```python
from build123d import *

# Parameters (mm, degrees)
F3_DEPTH  = 14
F5_DEPTH  = 5
F6_SIZE   = 2
F7_DEPTH  = 25
F9_DEPTH  = 51.6
F10_DEPTH = 1.1


# Not quite as in the source:
# - a feature names something its author has since deleted; it is built from what else it names


with BuildPart() as f3:
    # F2 (on line) → F3 (new body)
    with BuildSketch(Plane(origin=(0, 0, 0), x_dir=(0, 1, 0), z_dir=(0.984807753, 0, -0.1736481777))):
        with BuildLine():
            ThreePointArc((4.3133513652, 4.3133513652), (5.6356651483, 2.3343689374), (6.1, 0))
            ThreePointArc((6.1, 0), (-2.3343689374, -5.6356651483), (-4.3133513652, 4.3133513652))
            Line((-4.3133513652, 4.3133513652), (-6.4346717088, 6.4346717088))
            ThreePointArc((-6.4346717088, 6.4346717088), (-3.4824192345, -8.4073037459), (9.1, 0))
            ThreePointArc((9.1, 0), (8.4073037459, 3.4824192345), (6.4346717088, 6.4346717088))
            Line((6.4346717088, 6.4346717088), (4.3133513652, 4.3133513652))
        make_face()
    extrude(amount=F3_DEPTH)

    # F4 (on Front) → F5 (join, symmetric)
    with BuildSketch(Plane.XZ):
        Polygon((-0.9719453416, -8.4384017807), (-0.9719453416, -21.6384017807), (7.9780546584, -21.6384017807), (7.9780546584, -18.6384017807), (2.0280546584, -18.6384017807), (2.0280546584, -11.4384017807), (9.7280546584, -11.4384017807), (9.7280546584, -15.6384017807), (12.7280546584, -15.6384017807), (12.7280546584, -11.4438512443), (12.7280546584, -8.4384017807), align=None)
    extrude(amount=F5_DEPTH, both=True)

    # F6
    f6_edges = [f3.edges().sort_by_distance(p)[0] for p in [
        (9.728055, 0, -15.638402),
        (7.978055, 0, -18.638402),
    ]]
    chamfer(f6_edges, length=F6_SIZE)

    # F7 (add): a face of the model
    f7_faces = [f3.faces().sort_by_distance(p)[0] for p in [
        (-1.1008050308, 0, -6.2429755581),
    ]]
    extrude(f7_faces, amount=F7_DEPTH)

    # F8 (on face) → F9 (cut)
    with BuildSketch(Plane(origin=(-0.9719453416, 0, 0), x_dir=(0, -1, 0), z_dir=(-1, 0, 0))):
        with BuildLine():
            Line((22.6868242025, -11.5467039868), (22.6868242025, 11.5467039868))
            Line((22.6868242025, 11.5467039868), (-22.6868242025, 11.5467039868))
            Line((-22.6868242025, 11.5467039868), (-22.6868242025, -11.5467039868))
            Line((-22.6868242025, -11.5467039868), (-5, -11.5467039868))
            Line((-5, -11.5467039868), (-5, -8.4384017807))
            Line((-5, -8.4384017807), (-3.3040728779, -8.4384017807))
            add(Edge.make_bspline(
                [(-3.3040728779, -8.4384017807), (0, -9.7457887872), (3.3040728779, -8.4384017807)],
                knots=[2.7700160081, 2.7700160081, 2.7700160081, 3.5131692991, 3.5131692991, 3.5131692991], degree=2, weights=[1, 0.9317560477, 1]))
            Line((3.3040728779, -8.4384017807), (5, -8.4384017807))
            Line((5, -8.4384017807), (5, -11.5467039868))
            Line((5, -11.5467039868), (22.6868242025, -11.5467039868))
        make_face()
    extrude(amount=F9_DEPTH, mode=Mode.SUBTRACT)

    # F10 (add): faces of the model
    f10_faces = [f3.faces().sort_by_distance(p)[0] for p in [
        (0.6395749646, -4.4604313904, -8.4384017807),
        (0.6395749646, 4.4604313904, -8.4384017807),
    ]]
    extrude(f10_faces, amount=F10_DEPTH)


solid = f3.part
```
Verification items for the finished model (mm, model axes). A direction names the side the tool comes from. Round coordinates to 2 decimals unless told otherwise and drop trailing zeros. Loops run counter-clockwise (first coordinate to the right, second up) from the corner with the lowest first, then second, coordinate; pieces in that order, holes last. Notation, with made-up numbers: (-29, -39) -> (10, -39) arc R12 ccw to (10, -23) -> close; hole circle Ø10 at (50, 68.5). An arc over 180 degrees is marked (long way). Answer as a JSON object with one key per item and string values.
Q1. Section check B-B (y = -1.5). Record the boundary of the cut face in (x, z), then the cut area to 3 significant figures.
Data:
{"outline": "(-0.97, -21.64) -> (7.98, -21.64) -> (7.98, -20.64) -> (5.98, -18.64) -> (2.03, -18.64) -> (2.03, -11.44) -> (9.73, -11.44) -> (9.73, -13.64) -> (11.73, -15.64) -> (12.73, -15.64) -> (12.73, -8.44) -> (12.76, -8.25) -> (-0.97, -5.83) -> close", "area": "117 mm2"}
Q2. Access from +Z, -Z, +X, -X, +Y, -Y to the whole of each face (thin tool, end or side, straight path). Record for faces 5 (the flat face through (6.99, 0.07, -19.65)), 6 (the flat face through (7.978, 0, -21)), 7 (the flat face through (-0.972, 0, -10)), 8 (the flat face through (6.896, 5.389, 4.256)), 9 (the flat face through (6, 0, -11.438)).
Data:
{"face 5": "+X, +Y, -Y", "face 6": "-Z, +X, +Y, -Y", "face 7": "+Z, -Z, -X, +Y, -Y", "face 8": "+Z, +X", "face 9": "+Y, -Y"}
Q3. Draft check along X on faces 1 (the flat face through (9.728, 0, -13)), 2 (the flat face through (10.71, 0.07, -14.62)), 3 (the flat face through (12, 0, -15.638)), 4 (the flat face through (13.692, -6.593, -2.974)). Enter one of: pulls with the +X half, pulls with the -X half, needs draft (parallel to the pull), parting line crosses it, or undercut.
Data:
{"face 1": "undercut", "face 2": "undercut", "face 3": "needs draft", "face 4": "pulls with the +X half"}
Q4. Section check C-C (z = -18.25). Record the boundary of the cut face in (x, y).
Data:
{"outline": "(-0.97, -5) -> (2.03, -5) -> (2.03, 5) -> (-0.97, 5) -> close"}
Q5. Section check D-D (y = 2.25). Record the boundary of the cut face in (x, z), then the cut area to 3 significant figures.
Data:
{"outline": "(-0.97, -21.64) -> (7.98, -21.64) -> (7.98, -20.64) -> (5.98, -18.64) -> (2.03, -18.64) -> (2.03, -11.44) -> (9.73, -11.44) -> (9.73, -13.64) -> (11.73, -15.64) -> (12.73, -15.64) -> (12.73, -8.44) -> (12.8, -8.01) -> (-0.97, -5.59) -> close", "area": "121 mm2"}
Q6. Section check A-A (z = -12.75). Record the boundary of the cut face in (x, y).
Data:
{"outline": "(-0.97, -5) -> (2.03, -5) -> (2.03, 5) -> (-0.97, 5) -> close; (9.73, -5) -> (12.73, -5) -> (12.73, 5) -> (9.73, 5) -> close"}
Q7. Go/stop test with flat-tipped pins: P1, Ø6, axis at y = 2.5, z = -16.5, coming from the +X side; P2, Ø1.1, axis at x = 12.5, y = -2.5, coming from the -Z side; P3, Ø8, axis at y = 0, z = 3, coming from the -X side; P4, Ø3, axis at x = 3, y = 1.5, coming from the +Z side. Record where each tip stops, or that it passes through.
Data:
{"P1": "stops at x = 12.73", "P2": "stops at z = -15.64", "P3": "passes through", "P4": "stops at z = -5.88"}
Q8. Scan lines: line 1 (Y direction, x = 1, z = -16); line 2 (X direction, y = 1.5, z = -13); line 3 (X direction, y = -1.25, z = -17.5). Record each from-to range of solid material in increasing order. Write a range as from..to.
Data:
{"line 1": "y = -5..5", "line 2": "x = -0.97..2.03, 9.73..12.73", "line 3": "x = -0.97..2.03"}
